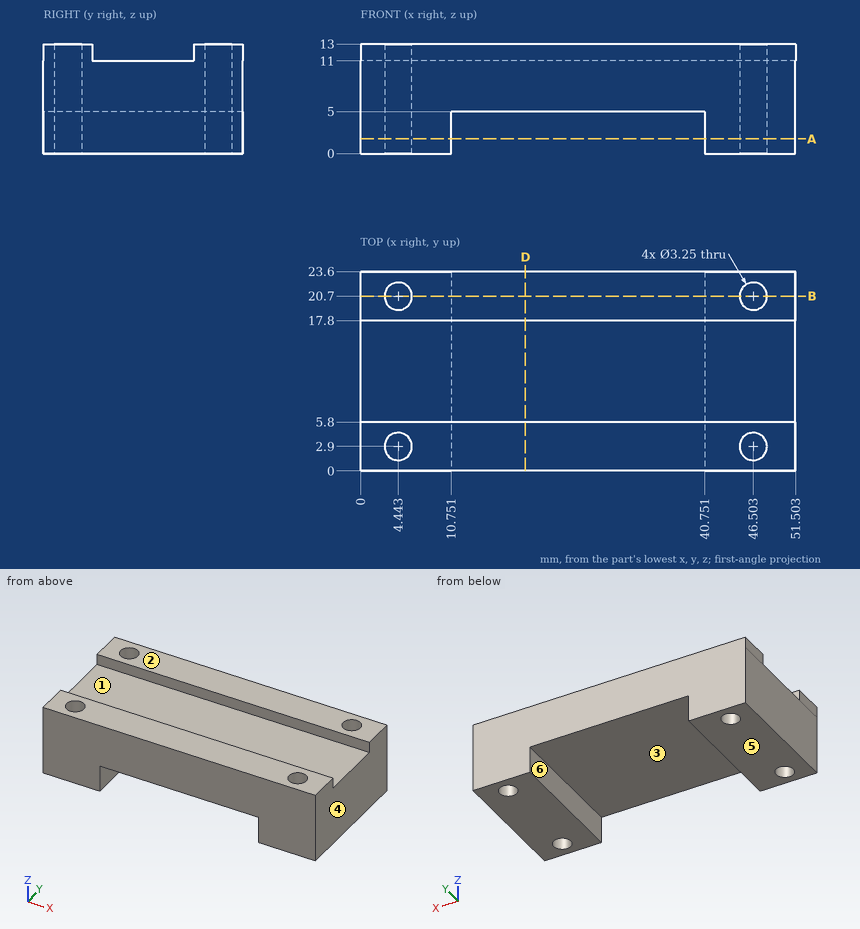
Geometry: see drawing. Coordinates: mm, zero at the bounding-box minimum. A direction names the side the tool comes from. Coordinates: 2 decimals unless noted, no trailing zeros. Loops run counter-clockwise (first coordinate to the right, second up) from the corner with the lowest first, then second, coordinate; pieces in that order, holes last.
Q1. Set-up query: the marked faces 1 and 2. Return all of +Z, -Z, +X, -X, +Y, -Y with unobstructed straight access to the full face (end or side cutting, diameter ignored); none if empty.
Q2. Cut plane D-D (x = 19.5). Output: boundary loops of the cut face in (y, z).
Q3. Material intervals for line 1 (X direction, y = 12.75, z = 2.5); line 2 (X direction, y = 22, z = 6.25) (1 decimal); line 3 (Z direction, x = 19, y = 9.5), sorted ascending.
Q4. Cut plane B-B (y = 20.7). Output: boundary loops of the cut face in (x, z), then the cut area to 3 significant figures.
Q5. Draft query along X for the marked faces 3, 4, 5 and 6. Return one class per face: +X half, -X half, draft (parallel to the pull), parting line (faces both ways), or undercut.
Q6. Cut plane A-A (z = 1.75). Give the number of separate pieces and of enclosed holes in the cut face, then the cut area to 3 significant figures.
Q7. Contact query for flat-ended pins moving along their axis: pin 1 (12 mm diameter, centred on x = 28.5, y = 15.5, fed in from -Z); pin 2 (3 mm diameter, centred on x = 4.44, y = 2.9, fed in from +Z); pin 3 (5 mm diameter, centred on x = 23.5, y = 12, fed in from +Z). Output: stop coordinate, or through.
Working result:
1. face 1: +Z, +X, -X
1. face 2: +Z, +X, -X, +Y, -Y
2. outline: (0, 5) - (23.6, 5) - (23.6, 13) - (17.8, 13) - (17.8, 11) - (5.8, 11) - (5.8, 13) - (0, 13) - close
3. line 1: x = 0 to 10.75, 40.75 to 51.5
3. line 2: x = 0 to 3.5, 5.4 to 45.5, 47.5 to 51.5
3. line 3: z = 5 to 11
4. outline: (0, 0) - (2.82, 0) - (2.82, 13) - (0, 13) - close; (6.07, 0) - (10.75, 0) - (10.75, 5) - (40.75, 5) - (40.75, 0) - (44.88, 0) - (44.88, 13) - (6.07, 13) - close; (48.13, 0) - (51.5, 0) - (51.5, 13) - (48.13, 13) - close
4. area: 435 mm2
5. face 3: undercut
5. face 4: +X half
5. face 5: draft
5. face 6: undercut
6. separate pieces: 2
6. enclosed holes: 4
6. area: 474 mm2
7. pin 1: stops at z = 5
7. pin 2: passes through
7. pin 3: stops at z = 11
